The model under review builds one solid part; all positions refer to its coordinate system, in mm. Give positions to 0.01 mm unless a question says otherwise; leave off trailing zeros. Order: outer loops, then holes, each group sorted by start corner. A loop starts at its lowest first (then second) coordinate and runs counter-clockwise, first axis right, second up. Notation, with made-up numbers: (28, 1) - (71, 1) arc R31 cw to (71, 31) - close; hole circle Ø1 at (18, -31.5). An arc over 180 degrees is marked (long way). Use CSV: the item, a comma, the result in double quotes.
Autodesk Inventor part; units mm, degrees
ref_plane "YZ Plane" through (0, 0, 0) normal (1, 0, 0) x (0, 1, 0)
ref_plane "XZ Plane" through (0, 0, 0) normal (0, 1, 0) x (-1, 0, 0)
ref_plane "XY Plane" through (0, 0, 0) normal (0, 0, 1) x (1, 0, 0)
sketch "Sketch1" plane through (0, 0, 0) normal (0, 0, 1) x (1, 0, 0)
  line L0 (3.6662, 6.35) -> (7.3323, 0)
  line L1 (7.3323, 0) -> (3.6662, -6.35)
  line L2 (3.6662, -6.35) -> (-3.6662, -6.35)
  line L3 (-3.6662, -6.35) -> (-7.3323, 0)
  line L4 (-7.3323, 0) -> (-3.6662, 6.35)
  line L5 (-3.6662, 6.35) -> (3.6662, 6.35)
  point P0 (0, 0)
  point P1 (0, 0)
  dimension "d0" = 12.7
extrude "Extrusion1" add sketch "Sketch1" along normal blind 177.8
properties part number "hex rod 7 inch" material "Steel, Alloy"
Item 1: Take a section at B-B, the plane y = 2.25. Give the boundary of the cut face in (x, z).
Results list:
outline,"(-6.03, 0) - (6.03, 0) - (6.03, 177.8) - (-6.03, 177.8) - close"
Item 2: Clearance check with flat-ended pins moving along their axes: pin 1 (1.5 mm diameter, centred on y = -4, z = 157, fed in from -X); pin 2 (6 mm diameter, centred on y = 2.5, z = 97.5, fed in from -X). State where each tip first meets the part, or that it passes through.
Results list:
pin 1,"stops at x = -5.46"
pin 2,"stops at x = -7.33"
Item 3: Wall thickness on L1, parallel to X at y = -4, z = 153; L2, parallel to Y at x = 4, z = 40; L3, parallel to X at y = -1.75, z = 135: over which ranges is each line inside the solid? List them lowest first.
Results list:
L1,"x = -5.02 to 5.02"
L2,"y = -5.77 to 5.77"
L3,"x = -6.32 to 6.32"
Item 4: Take a section at C-C, the plane y = -4.75. Give the boundary of the cut face in (x, z).
Results list:
outline,"(-4.59, 0) - (4.59, 0) - (4.59, 177.8) - (-4.59, 177.8) - close"
Item 5: Take a section at A-A, the plane z = 31. Give the boundary of the cut face in (x, y).
Results list:
outline,"(-7.33, 0) - (-3.67, -6.35) - (3.67, -6.35) - (7.33, 0) - (3.67, 6.35) - (-3.67, 6.35) - close"
